```python
from build123d import *

# Parameters (mm, degrees)
SKETCH1_W                                      = 165.1
SKETCH1_H                                      = 228.6
BOSS_EXTRUDE1_DEPTH                            = 12.7
SKETCH2_W                                      = 107.95
SKETCH2_H                                      = 203.2
CUT_EXTRUDE1_DEPTH                             = 142.563704741
SKETCH3_W                                      = 165.1
SKETCH3_H                                      = 9.525
BOSS_EXTRUDE2_DEPTH                            = 57.15
SKETCH4_W                                      = 19.05
SKETCH4_H                                      = 15.875
BOSS_EXTRUDE3_DEPTH                            = 12.7
CUT_EXTRUDE2_REACH                             = 159.347
SKETCH7_W                                      = 63.5
SKETCH7_H                                      = 12.7
BOSS_EXTRUDE4_DEPTH                            = 12.7
SKETCH8_W                                      = 57.15
SKETCH8_H                                      = 12.7
CUT_EXTRUDE4_DEPTH                             = 2.54
F_8_32_TAPPED_HOLE1_D                          = 3.4544
F_8_32_TAPPED_HOLE1_DEPTH                      = 12.7
F_8_32_TAPPED_HOLE1_TIP                        = 1.037806461
F_1_4_CLEARANCE_HOLE1_D                        = 6.7564
F_1_4_CLEARANCE_HOLE1_DEPTH                    = 10.16
F_6_32_TAPPED_HOLE2_D                          = 2.7051
F_1_4_28_TAPPED_HOLE1_D                        = 5.4102
CBORE_FOR_8_SOCKET_HEAD_CAP_SCREW1_D           = 4.4958
CBORE_FOR_8_SOCKET_HEAD_CAP_SCREW1_CBORE_D     = 7.9375
CBORE_FOR_8_SOCKET_HEAD_CAP_SCREW1_CBORE_DEPTH = 4.1656


with BuildPart() as part:
    # Sketch1 → Boss-Extrude1 (new body)
    with BuildSketch(Plane.XY):
        Rectangle(SKETCH1_W, SKETCH1_H)
    extrude(amount=BOSS_EXTRUDE1_DEPTH)

    # Sketch2 → Cut-Extrude1 (cut, through all)
    with BuildSketch(Plane.XY.offset(12.7)):
        with Locations((0, -12.7)):
            Rectangle(SKETCH2_W, SKETCH2_H)
    extrude(amount=-CUT_EXTRUDE1_DEPTH, mode=Mode.SUBTRACT)

    # Sketch3 → Boss-Extrude2 (add)
    with BuildSketch(Plane(origin=(0, 0, 0), x_dir=(-1, 0, 0), z_dir=(0, 0, -1))):
        with Locations((0, 109.5375)):
            Rectangle(SKETCH3_W, SKETCH3_H)
    extrude(amount=BOSS_EXTRUDE2_DEPTH)

    # Sketch4 → Boss-Extrude3 (add)
    with BuildSketch(Plane(origin=(0, 0, -57.15), x_dir=(-1, 0, 0), z_dir=(0, 0, -1))):
        with Locations((-73.025, 96.8375)):
            Rectangle(SKETCH4_W, SKETCH4_H)
    boss_extrude3 = extrude(amount=-BOSS_EXTRUDE3_DEPTH)

    # Mirror1: Boss-Extrude3 across plane
    add(boss_extrude3.mirror(Plane(origin=(0, 0, 0), x_dir=(0, 0, 1), z_dir=(1, 0, 0))))

    # Sketch5 → Cut-Extrude2 (cut, up to next)
    with BuildSketch(Plane(origin=(0, 0, -57.15), x_dir=(-1, 0, 0), z_dir=(0, 0, -1)), mode=Mode.PRIVATE) as cut_extrude2_sk1:
        Polygon((-72.503159889, 88.9), (-63.5, 90.4875), (-63.5, 88.9), align=None)
    cut_extrude2_tool1 = extrude(cut_extrude2_sk1.sketch, amount=-CUT_EXTRUDE2_REACH, mode=Mode.PRIVATE) & part.part
    cut_extrude2 = cut_extrude2_tool1.solids().sort_by_distance((66.501053, 89.429167, -57.15))[0]
    add(cut_extrude2, mode=Mode.SUBTRACT)

    # Mirror2: Cut-Extrude2 across plane
    add(cut_extrude2.mirror(Plane(origin=(0, 0, 0), x_dir=(0, 0, 1), z_dir=(1, 0, 0))), mode=Mode.SUBTRACT)

    # Sketch7 → Boss-Extrude4 (add)
    with BuildSketch(Plane.XY.offset(12.7)):
        with Locations((-68.2625, -107.95)):
            Rectangle(SKETCH7_W, SKETCH7_H)
    boss_extrude4 = extrude(amount=-BOSS_EXTRUDE4_DEPTH)

    # Sketch8 → Cut-Extrude4 (cut)
    with BuildSketch(Plane(origin=(0, -114.3, 0), x_dir=(-1, 0, 0), z_dir=(0, -1, 0))):
        with Locations((68.2625, -6.35)):
            Rectangle(SKETCH8_W, SKETCH8_H)
    cut_extrude4 = extrude(amount=-CUT_EXTRUDE4_DEPTH, mode=Mode.SUBTRACT)

    # Mirror3: Boss-Extrude4, Cut-Extrude4 across plane
    add(boss_extrude4.mirror(Plane(origin=(0, 0, 0), x_dir=(0, 0, 1), z_dir=(1, 0, 0))))
    add(cut_extrude4.mirror(Plane(origin=(0, 0, 0), x_dir=(0, 0, 1), z_dir=(1, 0, 0))), mode=Mode.SUBTRACT)

    # #8-32 Tapped Hole1
    with Locations(Plane(origin=(0, 114.3, 0), x_dir=(1, 0, 0), z_dir=(0, 1, 0))):
        with Locations((-76.2, -6.35), (-63.5, -6.35), (63.5, -6.35), (76.2, -6.35)):
            Hole(F_8_32_TAPPED_HOLE1_D / 2, depth=F_8_32_TAPPED_HOLE1_DEPTH)
            with Locations((0, 0, -(F_8_32_TAPPED_HOLE1_DEPTH + F_8_32_TAPPED_HOLE1_TIP / 2))):  # 118° drill point
                Cone(0, F_8_32_TAPPED_HOLE1_D / 2, F_8_32_TAPPED_HOLE1_TIP, mode=Mode.SUBTRACT)

    # 1/4 Clearance Hole1
    with Locations(Plane(origin=(0, -101.6, 0), x_dir=(1, 0, 0), z_dir=(0, 1, 0))):
        with Locations((-90.4875, -6.35), (-46.0375, -6.35), (46.0375, -6.35), (90.4875, -6.35)):
            Hole(F_1_4_CLEARANCE_HOLE1_D / 2, depth=F_1_4_CLEARANCE_HOLE1_DEPTH)

    # #6-32 Tapped Hole2 (through all)
    with Locations(Plane(origin=(0, 88.9, 0), x_dir=(-1, 0, 0), z_dir=(0, -1, 0))):
        with Locations((77.7875, 50.8), (68.2625, 50.8), (-77.7875, 50.8), (-68.2625, 50.8)):
            Hole(F_6_32_TAPPED_HOLE2_D / 2)

    # 1/4-28 Tapped Hole1 (through all)
    with Locations(Plane(origin=(0, 114.3, 0), x_dir=(1, 0, 0), z_dir=(0, 1, 0))):
        with Locations((0, 50.8)):
            Hole(F_1_4_28_TAPPED_HOLE1_D / 2)

    # CBORE for #8 Socket Head Cap Screw1 (through all)
    with Locations(Plane.XY.offset(12.7)):
        with Locations((-76.2, 34.925), (-60.325, 34.925), (60.325, 34.925), (76.2, 34.925)):
            CounterBoreHole(CBORE_FOR_8_SOCKET_HEAD_CAP_SCREW1_D / 2, CBORE_FOR_8_SOCKET_HEAD_CAP_SCREW1_CBORE_D / 2, CBORE_FOR_8_SOCKET_HEAD_CAP_SCREW1_CBORE_DEPTH)


solid = part.part
```
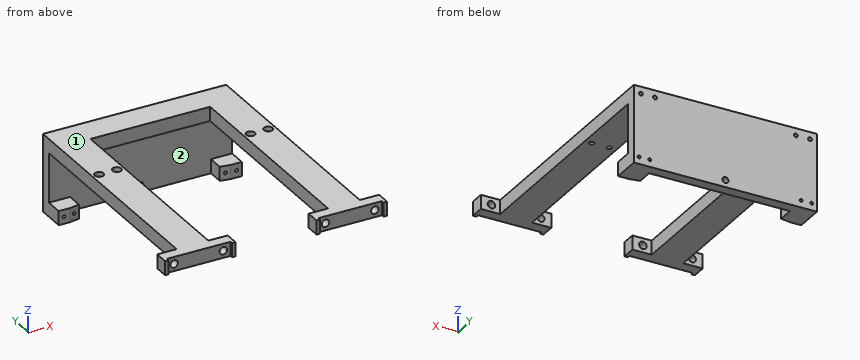
Model file for the job. Use its own axes, mm. Face numbers are marked on the shaded views. Round coordinates to 2 decimals unless told otherwise and drop trailing zeros. Write each loop counter-clockwise with the first axis right and the second up, starting at its lowest first coordinate (ties: lowest second). Pieces come first, ordered by that corner, then holes. Notation, with made-up numbers: M 71.5,-27 L 117.5,-27 A14 cw 117.5,-15 Z; hole C 21,62 d6. An arc over 180 degrees is marked long. Put each result on its own line as item: value.
Item 1: Probe L1, parallel to X at y = -105, z = 6; L2, parallel to X at y = -56, z = 4 (3 decimals); L3, parallel to X at y = 108.5, z = 6.35. List the from-to ranges inside material, lowest first. Write a range as from..to.
Responses:
L1: -100.01..-93.85, -87.13..-49.4, -42.68..-36.51, 36.51..42.68, 49.4..87.13, 93.85..100.01
L2: -82.55..-53.975, 53.975..82.55
L3: -82.55..-77.93, -74.47..-65.23, -61.77..61.77, 65.23..74.47, 77.93..82.55
Item 2: Mould opens along X. For the marked faces 1 and 2 say: +X half, -X half, draft (parallel to the pull), parting line (faces both ways), or undercut.
Responses:
face 1: draft
face 2: undercut
Item 3: Cut at A-A (y = 94). List the corners of the cut face in (x, z), and give its area (3 significant figures).
Responses:
outline: M -82.55,-57.15 L -63.5,-57.15 L -63.5,-44.45 L -82.55,-44.45 Z; M -82.55,0 L 82.55,0 L 82.55,12.7 L -82.55,12.7 Z; M 63.5,-57.15 L 82.55,-57.15 L 82.55,-44.45 L 63.5,-44.45 Z; hole C -77.79,-50.8 d2.71; hole C -68.26,-50.8 d2.71; hole C 68.26,-50.8 d2.71; hole C 77.79,-50.8 d2.71
area: 2,560 mm²
Item 4: Cut at B-B (y = 57). List the corners of the cut face in (x, z) (3 decimals).
Responses:
outline: M -82.55,0 L -53.975,0 L -53.975,12.7 L -82.55,12.7 Z; M 53.975,0 L 82.55,0 L 82.55,12.7 L 53.975,12.7 Z
Item 5: Flat gauge pins, fed straight in: P1, Ø4, axis at x = 63.5, z = 6.35, coming from the -Y side; P2, Ø10, axis at y = -42.5, z = 9, coming from the -X side; P3, Ø2, axis at x = -63.5, z = 6.35, coming from the +Y side. Where does each tip first touch, or does it go through?
Responses:
P1: y = -111.76
P2: x = -82.55
P3: y = 101.16
Item 6: Cut at D-D (x = -22). List the corners of the cut face in (y, z) (3 decimals).
Responses:
outline: M 88.9,0 L 104.775,0 L 104.775,-57.15 L 114.3,-57.15 L 114.3,12.7 L 88.9,12.7 Z
Item 7: Cut at C-C (x = 0). List the corners of the cut face in (y, z) (3 decimals).
Responses:
outline: M 88.9,0 L 104.775,0 L 104.775,-48.095 L 114.3,-48.095 L 114.3,12.7 L 88.9,12.7 Z; M 104.775,-57.15 L 114.3,-57.15 L 114.3,-53.505 L 104.775,-53.505 Z
